```python
from build123d import *
from OCP.BRepFilletAPI import BRepFilletAPI_MakeChamfer

# Parameters (mm, degrees)
SKETCH1_W           = 86
SKETCH1_H           = 45
SKETCH1_W_2         = 82
SKETCH1_H_2         = 41
BOSS_EXTRUDE1_DEPTH = 39.15
SKETCH2_W           = 86
SKETCH2_H           = 45
BOSS_EXTRUDE2_DEPTH = 2
BOSS_EXTRUDE3_DEPTH = 10
BOSS_EXTRUDE4_START = -5
BOSS_EXTRUDE4_DEPTH = 5
FILLET2_R           = 3
SKETCH5_W           = 35
SKETCH5_H           = 28
CUT_EXTRUDE1_DEPTH  = 5
BOSS_EXTRUDE5_REACH = 94.369
CHAMFER1_SIZE       = 8.660254038
CHAMFER1_SIZE_2     = 5
CHAMFER2_SIZE       = 6.551464217
CHAMFER2_SIZE_2     = 18
FILLET3_R           = 6
BOSS_EXTRUDE6_DEPTH = 2
BOSS_EXTRUDE7_DEPTH = 15


# Some blends are built 0.0001 mm under size
with BuildPart() as part:
    # Sketch1 → Boss-Extrude1 (new body)
    with BuildSketch(Plane.XY):
        Rectangle(SKETCH1_W, SKETCH1_H)
        Rectangle(SKETCH1_W_2, SKETCH1_H_2, mode=Mode.SUBTRACT)
    extrude(amount=-BOSS_EXTRUDE1_DEPTH)

    # Sketch2 → Boss-Extrude2 (add)
    with BuildSketch(Plane(origin=(0, 0, -39.15), x_dir=(-1, 0, 0), z_dir=(0, 0, -1))):
        Rectangle(SKETCH2_W, SKETCH2_H)
    extrude(amount=-BOSS_EXTRUDE2_DEPTH)

    # Sketch3 → Boss-Extrude3 (add)
    with BuildSketch(Plane(origin=(25, 0, 0), x_dir=(0, 0, -1), z_dir=(1, 0, 0))):
        with BuildLine():
            Line((69.527285586, 11.3), (69.527285586, 17.5))
            Line((69.527285586, 17.5), (39.15, 17.5))
            Line((39.15, 17.5), (39.15, -17.5))
            Line((39.15, -17.5), (69.527285586, -17.5))
            Line((69.527285586, -17.5), (69.527285586, -11.3))
            Line((69.527285586, -11.3), (59.527285586, -11.3))
            ThreePointArc((59.527285586, -11.3), (40.1, 0), (59.527285586, 11.3))
            Line((59.527285586, 11.3), (69.527285586, 11.3))
        make_face()
    extrude(amount=-BOSS_EXTRUDE3_DEPTH)

    # Sketch4 → Boss-Extrude4 (add)
    with BuildSketch(Plane.ZY.offset(25).offset(BOSS_EXTRUDE4_START)):
        with BuildLine():
            Line((-39.15, -17.5), (-39.15, 17.5))
            Line((-39.15, 17.5), (-69.527285586, 17.5))
            Line((-69.527285586, 17.5), (-69.527285586, 11.3))
            Line((-69.527285586, 11.3), (-59.527285586, 11.3))
            ThreePointArc((-59.527285586, 11.3), (-40.1, 0), (-59.527285586, -11.3))
            Line((-59.527285586, -11.3), (-69.527285586, -11.3))
            Line((-69.527285586, -11.3), (-69.527285586, -17.5))
            Line((-69.527285586, -17.5), (-39.15, -17.5))
        make_face()
    extrude(amount=BOSS_EXTRUDE4_DEPTH)

    # Fillet2
    fillet2_edges = [part.edges().sort_by_distance(p)[0] for p in [
        (20, -11.3, -69.527285586),
        (20, -17.5, -69.527285586),
        (20, -17.5, -39.15),
        (20, 17.5, -39.15),
        (20, 17.5, -69.527285586),
        (20, 11.3, -69.527285586),
        (-22.5, -17.5, -39.15),
        (-22.5, -17.5, -69.527285586),
        (-22.5, -11.3, -69.527285586),
        (-22.5, 11.3, -69.527285586),
        (-22.5, 17.5, -69.527285586),
        (-22.5, 17.5, -39.15),
    ]]
    fillet(fillet2_edges, radius=FILLET2_R)

    # Sketch5 → Cut-Extrude1 (cut)
    with BuildSketch(Plane(origin=(0, 0, -39.15), x_dir=(-1, 0, 0), z_dir=(0, 0, -1))):
        with Locations((2.5, 0)):
            Rectangle(SKETCH5_W, SKETCH5_H)
    extrude(amount=-CUT_EXTRUDE1_DEPTH, mode=Mode.SUBTRACT)

    # Boss-Extrude5: up to this face of the body (flat: up to its plane)
    boss_extrude5_end = Plane(part.part.faces().sort_by_distance((0, 20.5, -18.575))[0])
    # Sketch6 → Boss-Extrude5 (add, up to the picked face)
    with BuildSketch(Plane(origin=(0, -20.5, 0), x_dir=(1, 0, 0), z_dir=(0, 1, 0)), mode=Mode.PRIVATE) as boss_extrude5_sk1:
        Polygon((-20, 37.15), (-43, 28.778684612), (-43, 37.15), align=None)
    boss_extrude5_tool1 = split(extrude(boss_extrude5_sk1.sketch, amount=BOSS_EXTRUDE5_REACH, mode=Mode.PRIVATE), bisect_by=boss_extrude5_end, keep=Keep.BOTH, mode=Mode.PRIVATE)
    # Sketch6 → Boss-Extrude5 (add, up to the picked face)
    with BuildSketch(Plane(origin=(0, -20.5, 0), x_dir=(1, 0, 0), z_dir=(0, 1, 0)), mode=Mode.PRIVATE) as boss_extrude5_sk2:
        Polygon((15, 37.15), (43, 37.15), (43, 28.778684612), align=None)
    boss_extrude5_tool2 = split(extrude(boss_extrude5_sk2.sketch, amount=BOSS_EXTRUDE5_REACH, mode=Mode.PRIVATE), bisect_by=boss_extrude5_end, keep=Keep.BOTH, mode=Mode.PRIVATE)
    add(boss_extrude5_tool1.solids().sort_by(Axis((-35.333333, -20.5, -34.359562), (0, 1, 0)))[0])
    add(boss_extrude5_tool2.solids().sort_by(Axis((33.666667, -20.5, -34.359562), (0, 1, 0)))[0])

    # Chamfer1
    # the kernel refuses this chamfer: 8.660254038, 5 mm, written as the material it adds along each edge
    with BuildSketch(Plane(origin=(-42.404819853, 20.5, -37.15), x_dir=(0, -0.999813220622208, -0.019326765612700494), z_dir=(1, 0, 0))) as chamfer1_piece_1_section:
        Polygon((CHAMFER1_SIZE * 0.999813220604, -CHAMFER1_SIZE * 0.0193267656124), (-CHAMFER1_SIZE_2 * 0.0193267656127, -CHAMFER1_SIZE_2 * 0.999813220622), (0, 0), align=None)
    chamfer1_piece_1 = extrude(amount=79.809639706, mode=Mode.PRIVATE)
    chamfer1_piece_1 = split(chamfer1_piece_1, bisect_by=Plane(origin=(-20, 13.459936491, -36.526388375), z_dir=(-1, 0, 0)), keep=Keep.TOP, mode=Mode.PRIVATE)
    add(chamfer1_piece_1)
    with BuildSketch(Plane(origin=(-42.404819853, 20.5, -37.15), x_dir=(0, -0.999813220622208, -0.019326765612700494), z_dir=(1, 0, 0))) as chamfer1_piece_2_section:
        Polygon((CHAMFER1_SIZE * 0.999813220604, -CHAMFER1_SIZE * 0.0193267656124), (-CHAMFER1_SIZE_2 * 0.0193267656127, -CHAMFER1_SIZE_2 * 0.999813220622), (0, 0), align=None)
    chamfer1_piece_2 = extrude(amount=79.809639706, mode=Mode.PRIVATE)
    chamfer1_piece_2 = split(chamfer1_piece_2, bisect_by=Plane(origin=(-2.5, 14, -35.400332947), z_dir=(0, 1, 0)), keep=Keep.TOP, mode=Mode.PRIVATE)
    add(chamfer1_piece_2)
    with BuildSketch(Plane(origin=(-42.404819853, 20.5, -37.15), x_dir=(0, -0.999813220622208, -0.019326765612700494), z_dir=(1, 0, 0))) as chamfer1_piece_3_section:
        Polygon((CHAMFER1_SIZE * 0.999813220604, -CHAMFER1_SIZE * 0.0193267656124), (-CHAMFER1_SIZE_2 * 0.0193267656127, -CHAMFER1_SIZE_2 * 0.999813220622), (0, 0), align=None)
    chamfer1_piece_3 = extrude(amount=79.809639706, mode=Mode.PRIVATE)
    chamfer1_piece_3 = split(chamfer1_piece_3, bisect_by=Plane(origin=(15, 13.459936491, -36.526388375), z_dir=(1, 0, 0)), keep=Keep.TOP, mode=Mode.PRIVATE)
    add(chamfer1_piece_3)
    with BuildSketch(Plane(origin=(37.404819853, -20.5, -37.15), x_dir=(0, 0.999813220622208, -0.019326765612700494), z_dir=(-1, 0, 0))) as chamfer1_piece_4_section:
        Polygon((CHAMFER1_SIZE * 0.999813220604, -CHAMFER1_SIZE * 0.0193267656124), (-CHAMFER1_SIZE_2 * 0.0193267656127, -CHAMFER1_SIZE_2 * 0.999813220622), (0, 0), align=None)
    chamfer1_piece_4 = extrude(amount=79.809639706, mode=Mode.PRIVATE)
    chamfer1_piece_4 = split(chamfer1_piece_4, bisect_by=Plane(origin=(15, -13.459936491, -36.526388375), z_dir=(1, 0, 0)), keep=Keep.TOP, mode=Mode.PRIVATE)
    add(chamfer1_piece_4)
    with BuildSketch(Plane(origin=(37.404819853, -20.5, -37.15), x_dir=(0, 0.999813220622208, -0.019326765612700494), z_dir=(-1, 0, 0))) as chamfer1_piece_5_section:
        Polygon((CHAMFER1_SIZE * 0.999813220604, -CHAMFER1_SIZE * 0.0193267656124), (-CHAMFER1_SIZE_2 * 0.0193267656127, -CHAMFER1_SIZE_2 * 0.999813220622), (0, 0), align=None)
    chamfer1_piece_5 = extrude(amount=79.809639706, mode=Mode.PRIVATE)
    chamfer1_piece_5 = split(chamfer1_piece_5, bisect_by=Plane(origin=(-2.5, -14, -35.400332947), z_dir=(0, -1, 0)), keep=Keep.TOP, mode=Mode.PRIVATE)
    add(chamfer1_piece_5)
    with BuildSketch(Plane(origin=(37.404819853, -20.5, -37.15), x_dir=(0, 0.999813220622208, -0.019326765612700494), z_dir=(-1, 0, 0))) as chamfer1_piece_6_section:
        Polygon((CHAMFER1_SIZE * 0.999813220604, -CHAMFER1_SIZE * 0.0193267656124), (-CHAMFER1_SIZE_2 * 0.0193267656127, -CHAMFER1_SIZE_2 * 0.999813220622), (0, 0), align=None)
    chamfer1_piece_6 = extrude(amount=79.809639706, mode=Mode.PRIVATE)
    chamfer1_piece_6 = split(chamfer1_piece_6, bisect_by=Plane(origin=(-20, -13.459936491, -36.526388375), z_dir=(-1, 0, 0)), keep=Keep.TOP, mode=Mode.PRIVATE)
    add(chamfer1_piece_6)

    # Chamfer2
    chamfer2_edges_1 = [part.edges().sort_by_distance(p)[0] for p in [
        (-43, 0, -39.15),
    ]]
    chamfer2_side_1 = [part.faces().sort_by_distance(p)[0] for p in [
        (-43, 0, -39.018970716),
    ]]
    chamfer2_edges_2 = [part.edges().sort_by_distance(p)[0] for p in [
        (43, 0, -39.15),
    ]]
    chamfer2_side_2 = [part.faces().sort_by_distance(p)[0] for p in [
        (42.868970716, 0, -39.15),
    ]]
    chamfer2 = BRepFilletAPI_MakeChamfer(part.part.solid().wrapped)
    for e in chamfer2_edges_1:
        chamfer2.Add(CHAMFER2_SIZE - 0.0001, CHAMFER2_SIZE_2 - 0.0001, e.wrapped, chamfer2_side_1[0].wrapped)
    for e in chamfer2_edges_2:
        chamfer2.Add(CHAMFER2_SIZE_2 - 0.0001, CHAMFER2_SIZE - 0.0001, e.wrapped, chamfer2_side_2[0].wrapped)
    add(Compound.cast(chamfer2.Shape()), mode=Mode.REPLACE)  # a hair under: the kernel refuses the full size

    # Fillet3
    fillet3_edges = [part.edges().sort_by_distance(p)[0] for p in [
        (41, -20.5, -14.688317856),
        (41, 20.5, -14.688317856),
        (-41, 20.5, -14.75331254),
        (-41, -20.5, -14.75331254),
        (-43, -22.5, -16.299317891),
        (-43, 22.5, -16.299317891),
        (43, -22.5, -16.299317891),
        (43, 22.5, -16.299317891),
    ]]
    fillet(fillet3_edges, radius=FILLET3_R)

    # Sketch7 → Boss-Extrude6 (add)
    # profile 1 of 2: a face of its own
    with BuildSketch(Plane.XY):
        with BuildLine():
            Line((46, -16.5), (46, 16.5))
            ThreePointArc((46, 16.5), (43.363961031, 22.863961031), (37, 25.5))
            Line((37, 25.5), (-37, 25.5))
            ThreePointArc((-37, 25.5), (-43.363961031, 22.863961031), (-46, 16.5))
            Line((-46, 16.5), (-46, -16.5))
            ThreePointArc((-46, -16.5), (-43.363961031, -22.863961031), (-37, -25.5))
            Line((-37, -25.5), (37, -25.5))
            ThreePointArc((37, -25.5), (43.363961031, -22.863961031), (46, -16.5))
        make_face()
        with BuildLine():
            Line((37, 22.5), (-37, 22.5))
            ThreePointArc((-37, 22.5), (-41.242640687, 20.742640687), (-43, 16.5))
            Line((-43, 16.5), (-43, -16.5))
            ThreePointArc((-43, -16.5), (-41.242640687, -20.742640687), (-37, -22.5))
            Line((-37, -22.5), (37, -22.5))
            ThreePointArc((37, -22.5), (41.242640687, -20.742640687), (43, -16.5))
            Line((43, -16.5), (43, 16.5))
            ThreePointArc((43, 16.5), (41.242640687, 20.742640687), (37, 22.5))
        make_face(mode=Mode.SUBTRACT)
    # profile 2 of 2: a face of its own
    with BuildSketch(Plane.XY):
        with BuildLine():
            ThreePointArc((43, 16.5), (41.242640687, 20.742640687), (37, 22.5))
            Line((37, 22.5), (-37, 22.5))
            ThreePointArc((-37, 22.5), (-41.242640687, 20.742640687), (-43, 16.5))
            Line((-43, 16.5), (-43, -16.5))
            ThreePointArc((-43, -16.5), (-41.242640687, -20.742640687), (-37, -22.5))
            Line((-37, -22.5), (37, -22.5))
            ThreePointArc((37, -22.5), (41.242640687, -20.742640687), (43, -16.5))
            Line((43, -16.5), (43, 16.5))
        make_face()
        with BuildLine():
            ThreePointArc((35, 20.5), (39.242640687, 18.742640687), (41, 14.5))
            Line((41, 14.5), (41, -14.5))
            ThreePointArc((41, -14.5), (39.242640687, -18.742640687), (35, -20.5))
            Line((35, -20.5), (-35, -20.5))
            ThreePointArc((-35, -20.5), (-39.242640687, -18.742640687), (-41, -14.5))
            Line((-41, -14.5), (-41, 14.5))
            ThreePointArc((-41, 14.5), (-39.242640687, 18.742640687), (-35, 20.5))
            Line((-35, 20.5), (35, 20.5))
        make_face(mode=Mode.SUBTRACT)
    extrude(amount=BOSS_EXTRUDE6_DEPTH)

    # Sketch9 → Boss-Extrude7 (add)
    with BuildSketch(Plane(origin=(0, -7.5, 0), x_dir=(-1, 0, 0), z_dir=(0, -1, 0))):
        with BuildLine():
            ThreePointArc((44, 5.5), (43.707106781, 6.207106781), (43, 6.5))
            Line((43, 6.5), (43, 4.5))
            ThreePointArc((43, 4.5), (43.707106781, 4.792893219), (44, 5.5))
        make_face()
        with BuildLine():
            Line((43, 4.5), (43, 6.5))
            ThreePointArc((43, 6.5), (42, 5.5), (43, 4.5))
        make_face()
        with BuildLine():
            ThreePointArc((-43, 6.5), (-44, 5.5), (-43, 4.5))
            Line((-43, 4.5), (-43, 6.5))
        make_face()
        with BuildLine():
            Line((-43, 6.5), (-43, 4.5))
            ThreePointArc((-43, 4.5), (-42.292893219, 4.792893219), (-42, 5.5))
            ThreePointArc((-42, 5.5), (-42.292893219, 6.207106781), (-43, 6.5))
        make_face()
    extrude(amount=-BOSS_EXTRUDE7_DEPTH)


solid = part.part
```
Build history of the part. All positions in model axes, mm. A direction names the side the tool comes from. Give positions to 0.01 mm unless a question says otherwise; leave off trailing zeros. Loops run counter-clockwise (first coordinate to the right, second up) from the corner with the lowest first, then second, coordinate; pieces in that order, holes last.
1) 3-axis set-ups, long thin cutter, end or side, ignore diameter. For faces 5 (the face through (-2, -14, -38)), 6 (the face through (20, 17.5, -55)), 7 (the face through (41.289, -20.696, -17.148)), 8 (the face through (41.289, 20.696, -17.635)): which of +Z, -Z, +X, -X, +Y, -Y reach the whole face in a straight line?
Values follow:
face 5: +Z, -Z
face 6: -Z, +X, -X, +Y
face 7: -Z, +X, -Y
face 8: -Z, +X, +Y
2) Probe line 1 along X through (y, z) = (13, -50); line 2 along Y through (x, z) = (29.5, -5); line 3 along Y through (x, z) = (21.5, -53.1). List the from-to ranges inside material, lowest first.
Values follow:
line 1: x = -25 to -20, 15 to 25
line 2: y = -22.5 to -20.5, 20.5 to 22.5
line 3: y = -17.5 to -13, 13 to 17.5
3) Drop flat-ended pins along their axis: P1, Ø17, axis at x = 9.5, z = -12, coming from the -Y side; P2, Ø2, axis at x = 20, z = -62, coming from the +Y side; P3, Ø5, axis at y = 18, z = -35, coming from the +X side. Give the stop position or say it passes through.
Values follow:
P1: stops at y = -22.5
P2: stops at y = 17.5
P3: stops at x = 42.95
4) Band-saw the part on A-A on x = -7.5. List the corners of the cut face in (y, z).
Values follow:
outline: (-25.5, 0) - (-22.5, 0) - (-22.5, -39.15) - (-14, -39.15) - (-14, -35.9) - (-20.5, -32.15) - (-20.5, 2) - (-25.5, 2) - close; (14, -39.15) - (22.5, -39.15) - (22.5, 0) - (25.5, 0) - (25.5, 2) - (20.5, 2) - (20.5, -32.15) - (14, -35.9) - close
5) Band-saw the part on C-C on z = -14. List the corners of the cut face in (x, y).
Values follow:
outline: (-43, -16.5) arc R6 ccw to (-37, -22.5) - (37, -22.5) arc R6 ccw to (43, -16.5) - (43, 16.5) arc R6 ccw to (37, 22.5) - (-37, 22.5) arc R6 ccw to (-43, 16.5) - close; hole (-41, -14.5) arc R6 ccw to (-35, -20.5) - (35, -20.5) arc R6 ccw to (41, -14.5) - (41, 14.5) arc R6 ccw to (35, 20.5) - (-35, 20.5) arc R6 ccw to (-41, 14.5) - close
6) Band-saw the part on D-D on z = -53.1. List the corners of the cut face in (x, y), then the cut area to 3 significant figures.
Values follow:
outline: (-25, -17.5) - (-20, -17.5) - (-20, -13) - (-25, -13) - close; (-25, 13) - (-20, 13) - (-20, 17.5) - (-25, 17.5) - close; (15, -17.5) - (25, -17.5) - (25, -13) - (15, -13) - close; (15, 13) - (25, 13) - (25, 17.5) - (15, 17.5) - close
area: 135 mm2
7) Two-plate mould, pull along X, no slides. Class faces 1 (the face through (-2, 14, -38)), 2 (the face through (-22, -11.3, -63)), 3 (the face through (15, -3, -40)), 4 (the face through (-25, -12.1, -47.7)): released by +X, released by -X, zero draft, split by the parting line, or undercut.
Values follow:
face 1: undercut
face 2: zero draft
face 3: undercut
face 4: released by -X
